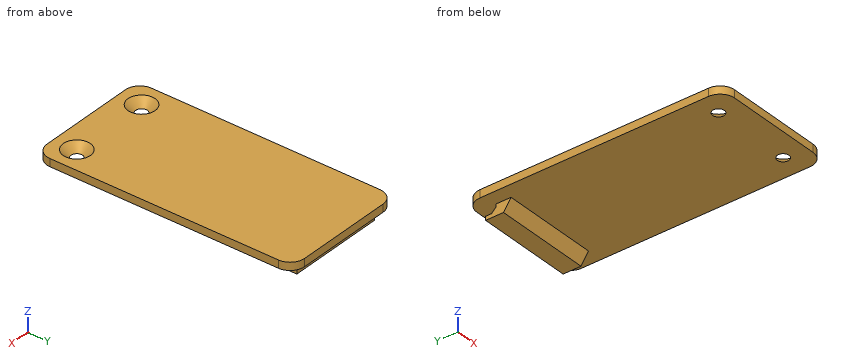
Autodesk Inventor part; units mm, degrees
ref_plane "Work Plane1" through (-10.1, -23.6, 0) normal (-1, 0, 0) x (0, 0, 1)
ref_plane "YZ Plane" through (0, 0, 0) normal (1, 0, 0) x (0, 1, 0)
ref_plane "XZ Plane" through (0, 0, 0) normal (0, 1, 0) x (-1, 0, 0)
sketch "Sketch1" plane through (0, 0, 0) normal (0, 0, 1) x (1, 0, 0)
  arc A0 (13.1, 23.6) -> (10.1, 26.6) centre (10.1, 23.6) ccw
  line L0 (10.1, 26.6) -> (-10.1, 26.6)
  arc A1 (-10.1, 26.6) -> (-13.1, 23.6) centre (-10.1, 23.6) ccw
  line L1 (-13.1, 23.6) -> (-13.1, -23.6)
  arc A2 (-13.1, -23.6) -> (-10.1, -26.6) centre (-10.1, -23.6) ccw
  line L2 (-10.1, -26.6) -> (10.1, -26.6)
  arc A3 (10.1, -26.6) -> (13.1, -23.6) centre (10.1, -23.6) ccw
  line L3 (13.1, -23.6) -> (13.1, 23.6)
  line L4 (11.5, 23) -> (11.5, -21.8566)
  line L5 (11.5, -21.8566) -> (11.5, -25)
  line L6 (11.5, -25) -> (8.3566, -25)
  line L7 (8.3566, -25) -> (-8.3566, -25)
  line L8 (-8.3566, -25) -> (-11.5, -25)
  line L9 (-11.5, -25) -> (-11.5, -21.8566)
  line L10 (-11.5, -21.8566) -> (-11.5, 23)
  line L11 (11.5, 23) -> (-11.5, 23)
  point P0 (0, 0)
extrude "Extrusion1" add sketch "Sketch1" along normal blind 1.6 contours L3 A3 L2 A2 L1 A1 L0 A0 | L4 L5 L6 L7 L8 L9 L10 L11
sketch "Sketch2" plane through (0, 0, 0) normal (0, 0, -1) x (-1, 0, 0)
  circle A0 centre (8.3566, -21.8566) radius 1.2
  circle A1 centre (-8.3566, -21.8566) radius 1.2
  point P0 (0, 0)
extrude "Extrusion2" cut sketch "Sketch2" against normal blind 1.6
chamfer "Chamfer1" distance 1.6 angle 45 2 edges at (9.5566, -21.8566, 1.6) (-7.1566, -21.8566, 1.6)
sketch "Sketch3" plane through (0, 0, 0) normal (0, 0, -1) x (-1, 0, 0)
  circle A0 centre (8.3566, -21.8566) radius 1.2
  circle A1 centre (-8.3566, -21.8566) radius 1.2
  arc A2 (-10.1, 26.6) -> (-13.1, 23.6) centre (-10.1, 23.6) ccw
  line L0 (-13.1, 23.6) -> (-13.1, -23.6)
  arc A3 (-13.1, -23.6) -> (-10.1, -26.6) centre (-10.1, -23.6) ccw
  line L1 (-10.1, -26.6) -> (10.1, -26.6)
  arc A4 (10.1, -26.6) -> (13.1, -23.6) centre (10.1, -23.6) ccw
  line L2 (13.1, -23.6) -> (13.1, 23.6)
  arc A5 (13.1, 23.6) -> (10.1, 26.6) centre (10.1, 23.6) ccw
  line L3 (10.1, 26.6) -> (-10.1, 26.6)
  point P0 (0, 0)
sketch "Sketch6" plane through (-13.1, -23.6, 1.6) normal (-1, 0, 0) x (0, 0, 1)
  line L0 (-1.6, 0) -> (-1.6, 47.2)
  line L1 (-1.6, 46.2477) -> (-2.136, 46.2477)
  line L2 (-2.136, 46.2477) -> (-3.0883, 47.2)
  line L3 (-3.0883, 47.2) -> (-3.0883, 48.4263)
  line L4 (-3.0883, 48.4263) -> (-3.8887, 48.4263)
  line L5 (-3.8887, 48.4263) -> (-3.8887, 44.7406)
  line L6 (-3.8887, 44.7406) -> (-1.6, 43.1845)
  line L7 (-1.6, 46.2477) -> (-1.6, 43.1845)
  point P0 (-1.6, 23.6)
  point P1 (-1.6, 1.7434)
extrude "Extrusion4" cut sketch "Sketch6" against normal blind 3
sketch "Sketch7" plane through (13.1, -23.6, 1.6) normal (1, 0, 0) x (0, 0, -1)
  line L0 (3.8887, 44.7406) -> (1.6, 43.1845)
  line L1 (3.8887, 48.4263) -> (3.8887, 44.7406)
  line L2 (3.0883, 48.4263) -> (3.8887, 48.4263)
  line L3 (3.0883, 47.2) -> (3.0883, 48.4263)
  line L4 (2.136, 46.2477) -> (3.0883, 47.2)
  line L5 (1.6, 46.2477) -> (2.136, 46.2477)
  line L6 (1.6, 46.2477) -> (1.6, 43.1845)
  point P0 (1.6, 23.6)
extrude "Extrusion5" cut sketch "Sketch7" against normal blind 3
ref_plane "Work Plane1" through (-10.1, -23.6, 0) normal (-1, 0, 0) x (0, 0, 1)
sketch "Sketch8" plane through (-10.1, -23.6, 0) normal (-1, 0, 0) x (0, 0, 1)
  line L0 (-0.536, 46.2477) -> (-1.4883, 47.2)
  line L1 (-1.4883, 47.2) -> (-1.4883, 48.4263)
  line L2 (-1.4883, 48.4263) -> (-2.2887, 48.4263)
  line L3 (-2.2887, 48.4263) -> (-2.2887, 44.7406)
  line L4 (-2.2887, 44.7406) -> (0, 43.1845)
  line L5 (0, 46.2477) -> (-0.536, 46.2477)
  line L6 (0, 0) -> (0, 47.2)
  point P0 (0, 23.6)
extrude "Extrusion6" add sketch "Sketch8" against normal blind 20
properties part number "top v3"
Check sheet for the modelled part. Datum: model origin and axes. Units: mm. Round coordinates to 2 decimals unless told otherwise and drop trailing zeros. Loops run counter-clockwise (first coordinate to the right, second up) from the corner with the lowest first, then second, coordinate; pieces in that order, holes last. Notation, with made-up numbers: M -5.75,37 L 16.25,37 A20 ccw 16.25,43 Z; hole C 58.5,52 d6. An arc over 180 degrees is marked long. Answer as a JSON object with one key per item and string values.
1. Gauge pin test, flat ends, axial feed: P1, Ø13, axis at x = 5, y = 2, coming from the -Z side; P2, Ø1.8, axis at y = 21.5, z = -1, coming from the +X side; P3, Ø0.6, axis at x = 2.5, z = -1.5, coming from the +Y side; P4, Ø1.9, axis at x = 8.36, y = -21.86, coming from the +Z side. Record the tip position at first contact, or that the pin passes through.
Reply:
{"P1": "stops at z = 0", "P2": "stops at x = 9.9", "P3": "stops at y = 24.83", "P4": "passes through"}
2. Section check C-C (y = 4). Record the boundary of the cut face in (x, z).
Reply:
{"outline": "M -13.1,0 L 13.1,0 L 13.1,1.6 L -13.1,1.6 Z"}
3. Scan lines: line 1 (X direction, y = -23, z = 1.4); line 2 (Z direction, x = -11.25, y = -6); line 3 (Y direction, x = -8.25, z = 1.3). Record each from-to range of solid material in increasing order.
Reply:
{"line 1": "x = -13.1 to -10.69, -6.02 to 6.02, 10.69 to 13.1", "line 2": "z = 0 to 1.6", "line 3": "y = -26.6 to -24.35, -19.36 to 26.6"}
4. Section check B-B (z = 1). Record the boundary of the cut face in (x, y).
Reply:
{"outline": "M -13.1,-23.6 A3 ccw -10.1,-26.6 L 10.1,-26.6 A3 ccw 13.1,-23.6 L 13.1,23.6 A3 ccw 10.1,26.6 L -10.1,26.6 A3 ccw -13.1,23.6 Z; hole C -8.36,-21.86 d4.4; hole C 8.36,-21.86 d4.4"}
5. Section check A-A (x = 0.75). Record the boundary of the cut face in (y, z).
Reply:
{"outline": "M -26.6,0 L 19.58,0 L 21.14,-2.29 L 24.83,-2.29 L 24.83,-1.49 L 23.6,-1.49 L 22.65,-0.54 L 22.65,0 L 26.6,0 L 26.6,1.6 L -26.6,1.6 Z"}
